Read the model definition and answer for the solid it produces. Units are mm, in the model's axes. Give positions to 0.01 mm unless a question says otherwise; leave off trailing zeros. Order: outer loops, then holes, each group sorted by start corner. A loop starts at its lowest first (then second) coordinate and runs counter-clockwise, first axis right, second up. Notation, with made-up numbers: M 34,66 L 90,66 A14 cw 90,89 Z; hole C 76.25,49 d2. An arc over 180 degrees is marked long. One line per item, written item: value. Start each with the question number.
from build123d import *

# Parameters (mm, degrees)
CROQUIS1_W              = 182
CROQUIS1_H              = 182
SALIENTE_EXTRUIR1_DEPTH = 2
CROQUIS2_R              = 4
CORTAR_EXTRUIR1_DEPTH   = 4


with BuildPart() as part:
    # Croquis1 → Saliente-Extruir1 (new, symmetric)
    with BuildSketch(Plane.XY):
        with Locations((91, 91)):
            Rectangle(CROQUIS1_W, CROQUIS1_H)
    extrude(amount=SALIENTE_EXTRUIR1_DEPTH, both=True)

    # Croquis2 → Cortar-Extruir1 (cut)
    with BuildSketch(Plane.XY.offset(2)):
        with Locations((30, 152)):
            Circle(CROQUIS2_R)
        with Locations((152, 152)):
            Circle(CROQUIS2_R)
        with Locations((152, 30)):
            Circle(CROQUIS2_R)
        with Locations((30, 30)):
            Circle(CROQUIS2_R)
    extrude(amount=-CORTAR_EXTRUIR1_DEPTH, mode=Mode.SUBTRACT)


solid = part.part
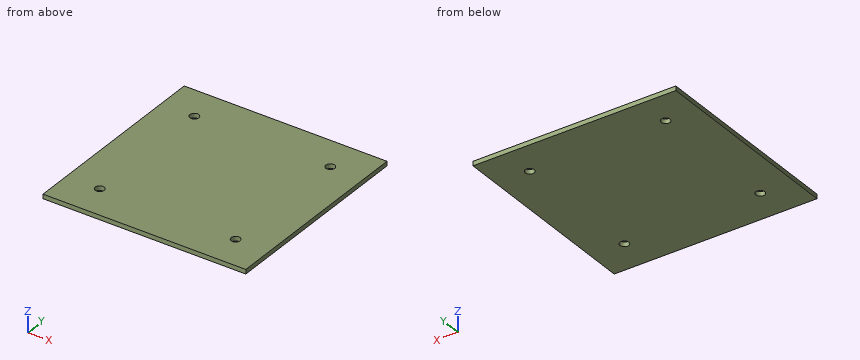
Q1. This flat-tipped pin is pushed along its axis until it touches: pin 1 (6.5 mm diameter, centred on x = 152, y = 152, fed in from -Z). Where does it stop, or does it pass through?
Q2. Find section A-A, the plane x = 30. Give the vertices of the cut face in (y, z).
Q3. Consider probe 1 along Y at (x, z) = (152, 0.7); probe 2 along X at (y, z) = (28, 1.55). Determine where each line is inside the solid, lowest interval first.
Evaluation:
1. pin 1: through
2. outline: M 0,-2 L 26,-2 L 26,2 L 0,2 Z; M 34,-2 L 148,-2 L 148,2 L 34,2 Z; M 156,-2 L 182,-2 L 182,2 L 156,2 Z
3. probe 1: 0 to 26, 34 to 148, 156 to 182
3. probe 2: 0 to 26.54, 33.46 to 148.54, 155.46 to 182
